The listing builds one solid part. Answer for the finished solid, in the listing's coordinates (mm). Face numbers are marked on the shaded views. Coordinates: 2 decimals unless noted, no trailing zeros. Order: outer loops, then holes, each group sorted by start corner. A loop starts at its lowest first (then second) coordinate and runs counter-clockwise, first axis right, second up. Notation, with made-up numbers: (55, 78.5) -> (82, 78.5) arc R29 ccw to (82, 114.5) -> close; hole circle Ø6 at (-12, -5). An arc over 180 degrees is marked (long way). Answer in a Markdown table with one row per item. Add a question column.
```python
from build123d import *

# Parameters (mm, degrees)
F1_DEPTH = 5
F5_DEPTH = 7
F6_DEPTH = 7
F7_DEPTH = 20
F8_R     = 1.75
F9_DEPTH = 25
F10_R    = 1


with BuildPart() as f1:
    # F0 (on Top) → F1 (new body)
    with BuildSketch(Plane.XY):
        Polygon((20, 0), (0, 0), (-10, 0), (-10, -3), (-2.5, -3), (0, -3), (20.5, -3), (23.5, -3), (30, -3), (30, 0), align=None)
    extrude(amount=F1_DEPTH)

    # F4 (on offset) → F5 (join)
    with BuildSketch(Plane.YZ.offset(10)):
        with BuildLine():
            ThreePointArc((-20.146994, 9.90317), (-20.877413, 10.144748), (-21.563228, 9.796137))
            ThreePointArc((-21.563228, 9.796137), (-18.370933, -7.385119), (-2.218958, -0.714286))
            ThreePointArc((-2.218958, -0.714286), (-1.858257, -0.198216), (-1.260643, 0))
            Line((-1.260643, 0), (0, 0))
            Line((0, 0), (0, 5))
            Line((0, 5), (-1.260643, 5))
            ThreePointArc((-1.260643, 5), (-1.858257, 5.198216), (-2.218958, 5.714286))
            ThreePointArc((-2.218958, 5.714286), (-2.524724, 6.602571), (-2.903535, 7.462248))
            ThreePointArc((-2.903535, 7.462248), (-3.517026, 7.979991), (-4.313516, 7.879836))
            ThreePointArc((-4.313516, 7.879836), (-4.745518, 7.30587), (-4.681243, 6.590376))
            ThreePointArc((-4.681243, 6.590376), (-14.149841, -6.698411), (-20.055883, 8.512273))
            ThreePointArc((-20.055883, 8.512273), (-19.819174, 9.226211), (-20.146994, 9.90317))
        make_face()
    extrude(amount=-F5_DEPTH)

    # F4 (on offset) → F6 (join)
    with BuildSketch(Plane.YZ.offset(10)):
        with BuildLine():
            ThreePointArc((-20.146994, 9.90317), (-20.877413, 10.144748), (-21.563228, 9.796137))
            ThreePointArc((-21.563228, 9.796137), (-18.370933, -7.385119), (-2.218958, -0.714286))
            ThreePointArc((-2.218958, -0.714286), (-1.858257, -0.198216), (-1.260643, 0))
            Line((-1.260643, 0), (0, 0))
            Line((0, 0), (0, 5))
            Line((0, 5), (-1.260643, 5))
            ThreePointArc((-1.260643, 5), (-1.858257, 5.198216), (-2.218958, 5.714286))
            ThreePointArc((-2.218958, 5.714286), (-2.524724, 6.602571), (-2.903535, 7.462248))
            ThreePointArc((-2.903535, 7.462248), (-3.517026, 7.979991), (-4.313516, 7.879836))
            ThreePointArc((-4.313516, 7.879836), (-4.745518, 7.30587), (-4.681243, 6.590376))
            ThreePointArc((-4.681243, 6.590376), (-14.149841, -6.698411), (-20.055883, 8.512273))
            ThreePointArc((-20.055883, 8.512273), (-19.819174, 9.226211), (-20.146994, 9.90317))
        make_face()
    extrude(amount=F6_DEPTH)

    # F0 (on Top) → F7 (join)
    with BuildSketch(Plane.XY):
        Polygon((20, 0), (0, 0), (-10, 0), (-10, -3), (-2.5, -3), (0, -3), (20.5, -3), (23.5, -3), (30, -3), (30, 0), align=None)
    extrude(amount=F7_DEPTH)

    # F8 (on face) → F9 (cut)
    with BuildSketch(Plane.XZ.offset(3)):
        with Locations((-5, 10)):
            Circle(F8_R)
        with Locations((25, 10)):
            Circle(F8_R)
    extrude(amount=-F9_DEPTH, mode=Mode.SUBTRACT)

    # F10
    f10_edges = [f1.edges().sort_by_distance(p)[0] for p in [
        (10, -3, 20),
        (30, -3, 10),
        (-10, -3, 10),
        (-6.75, -3, 10),
        (23.25, -3, 10),
    ]]
    fillet(f10_edges, radius=F10_R)


solid = f1.part
```
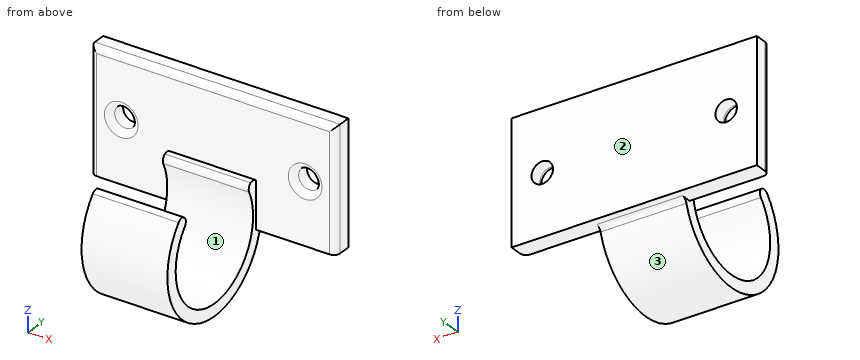
Q1. A cutting plane is placed at C-C (x = 6). Determine the outline of the cut face in (y, z).
Q2. Determine the mould class of the marked faces 1, 2 and 3 for opening direction Y: +Y half, -Y half, draft (parallel to the pull), parting line (faces both ways), or undercut.
Q3. A cutting plane is placed at A-A (z = 2.5). Determine the outline of the cut face in (x, y).
Q4. A cutting plane is placed at D-D (z = 16). Determine the outline of the cut face in (x, y), then the cut area to 3 significant figures.
Q5. Straight lines are drawn through the part: line 1 (Z direction, x = -5, y = -1.6); line 2 (Y direction, x = 28, z = 2.75); line 3 (X direction, y = -6, z = -6.25). For each, find the intervals that lie inside material, in ascending order.
Q6. A cutting plane is placed at B-B (x = 25). Determine the outline of the cut face in (y, z), then the cut area to 3 significant figures.
Q7. Given pin 1 (5.5 mm diameter, centred on x = 25, z = 10, fed in from +Y); pin 2 (9.5 mm diameter, centred on x = 12, z = 7.5, fed in from -Y); pin 3 (6 mm diameter, centred on x = 15.5, y = -5.5, fed in from +Z), each flat-ended and moving along its own axis, determine where each tip first touches the part or whether it passes through.
Returned:
| question | item | result |
|---|---|---|
| 1 | outline | (-21.56, 9.8) arc R11.25 ccw (long way) to (-2.22, -0.71) arc R1 cw to (-1.26, 0) -> (0, 0) -> (0, 20) -> (-2, 20) arc R1 ccw to (-3, 19) -> (-3, 7.62) arc R1 ccw to (-4.31, 7.88) arc R1 ccw to (-4.68, 6.59) arc R9.27 cw (long way) to (-20.06, 8.51) arc R1 ccw to (-20.15, 9.9) arc R1 ccw to start |
| 2 | face 1 | undercut |
| 2 | face 2 | +Y half |
| 2 | face 3 | parting line |
| 3 | outline | (-10, -2) arc R1 ccw to (-9, -3) -> (3, -3) -> (3, -3.73) -> (17, -3.73) -> (17, -3) -> (29, -3) arc R1 ccw to (30, -2) -> (30, 0) -> (-10, 0) -> close; (3, -24.25) -> (17, -24.25) -> (17, -22.27) -> (3, -22.27) -> close |
| 4 | outline | (-10, -2) arc R1 ccw to (-9, -3) -> (29, -3) arc R1 ccw to (30, -2) -> (30, 0) -> (-10, 0) -> close |
| 4 | area | 120 mm² |
| 5 | line 1 | z = 0 to 8.25, 11.75 to 20 |
| 5 | line 2 | y = -3 to 0 |
| 5 | line 3 | x = 3 to 17 |
| 6 | outline | (-3, 0) -> (0, 0) -> (0, 8.25) -> (-2, 8.25) arc R1 ccw to (-3, 7.25) -> close; (-3, 12.75) arc R1 ccw to (-2, 11.75) -> (0, 11.75) -> (0, 20) -> (-2, 20) arc R1 ccw to (-3, 19) -> close |
| 6 | area | 48.9 mm² |
| 7 | pin 1 | stops at y = 0 |
| 7 | pin 2 | stops at y = -24.25 |
| 7 | pin 3 | stops at z = 19.87 |
